Model file for the job. Use its own axes, mm. Face numbers are marked on the shaded views. A direction names the side the tool comes from. Round coordinates to 2 decimals unless told otherwise and drop trailing zeros. Return JSON: item names as keys, results as strings. Group by question number.
Item 1: Probe line 1 along X through (y, z) = (56, 29); line 2 along Z through (x, y) = (82.5, -83.5) (3 decimals); line 3 along X through (y, z) = (40.5, 4). List the from-to ranges inside material, lowest first.
Item 2: Which spindle directions (+Z, -Z, +X, -X, +Y, -Y) get a long thin tool onto all of the face, cutting with end or side? Do the marked faces 4, 5 and 6. Say none if no direction does.
Item 3: Slice it at A-A on z = 25.5. Give the number of separate pieces and of enclosed holes in the cut face, then the cut area to 3 significant figures.
Item 4: Pin check, flat tips, straight feed: pin 1 Ø5 at (x, y) = (-50.5, 11) entering from -Z; pin 2 Ø12 at (y, z) = (-56, 22) entering from +X; pin 3 Ø20.5 at (y, z) = (-71, 27) entering from -X. Stop position of each tip, or through.
Item 5: Pull direction X, two halves, no side cores. Call the marked faces 1, 2 and 3: pulls with the +X half, pulls with the -X half, needs draft (parallel to the pull), parting line crosses it, or undercut.
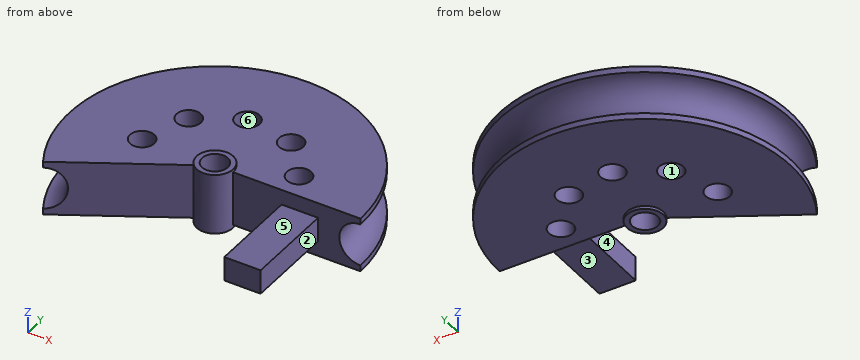
from build123d import *

# Parameters (mm, degrees)
F1_ANGLE = 210
F2_R     = 13.49375
F3_DEPTH = 69.85
F4_R     = 12.7
F5_DEPTH = 63.5
F6_W     = 38.1
F6_H     = 25.4
F7_DEPTH = 95.25
F8_R     = 19.05
F8_R_2   = 13.49375
F9_DEPTH = 63.5


with BuildPart() as f1:
    # F0 (on Front) → F1 (revolve)
    with BuildSketch(Plane.XZ):
        with BuildLine():
            Line((19.05, 57.15), (19.05, 0))
            Line((19.05, 0), (152.4, 0))
            Line((152.4, 0), (152.4, 6.35))
            ThreePointArc((152.4, 6.35), (130.175, 28.575), (152.4, 50.8))
            Line((152.4, 50.8), (152.4, 57.15))
            Line((152.4, 57.15), (19.05, 57.15))
        make_face()
        Polygon((19.05, -3.175), (19.05, 0), (19.05, 57.15), (19.05, 60.325), (0, 60.325), (0, 57.15), (0, 0), (0, -3.175), align=None)
    revolve(axis=Axis((0, 0, 28.575), (0, 0, 1)), revolution_arc=F1_ANGLE)

    # F2 (on face) → F3 (cut)
    with BuildSketch(Plane.XY.offset(60.325)):
        Circle(F2_R)
    extrude(amount=-F3_DEPTH, mode=Mode.SUBTRACT)

    # F4 (on face) → F5 (cut)
    with BuildSketch(Plane.XY.offset(57.15)):
        with Locations((-76.2, 0)):
            Circle(F4_R)
        with Locations((-58.372587, 48.980416)):
            Circle(F4_R)
        with Locations((-13.231991, 75.042351)):
            Circle(F4_R)
        with Locations((38.1, 65.991136)):
            Circle(F4_R)
        with Locations((71.604578, 26.061935)):
            Circle(F4_R)
    extrude(amount=-F5_DEPTH, mode=Mode.SUBTRACT)

    # F6 (on face) → F7 (join)
    with BuildSketch(Plane.XZ):
        with Locations((88.9, 28.575)):
            Rectangle(F6_W, F6_H)
    extrude(amount=F7_DEPTH)

    # F8 (on face) → F9 (join)
    with BuildSketch(Plane.XY.offset(60.325)):
        Circle(F8_R)
        Circle(F8_R_2, mode=Mode.SUBTRACT)
    extrude(amount=-F9_DEPTH)


solid = f1.part
Output values:
{
 "1": {"line 1": "-117.52 to -68.96, -47.79 to 30.26, 45.94 to 117.52", "line 2": "15.875 to 41.275", "line 3": "-146.92 to -67.83, -48.92 to 146.92"},
 "2": {"face 4": "+Z, -Z, -Y", "face 5": "+Z, +X, -Y", "face 6": "+Z, -Z"},
 "3": {"separate pieces": "1", "enclosed holes": "6", "area": "32,200 mm²"},
 "4": {"pin 1": "z = 0", "pin 2": "x = 107.95", "pin 3": "x = -115.61"},
 "5": {"face 1": "undercut", "face 2": "pulls with the +X half", "face 3": "needs draft"}
}
